Study the drawing (mm; zero at the part's minimum x, y, z) and answer. A direction names the side the tool comes from. Give positions to 0.01 mm unless a question says otherwise; leave off trailing zeros. Write each loop counter-clockwise with the first axis right and the second up, starting at its lowest first coordinate (ties: lowest second). Pieces come first, ordered by that corner, then holes. Notation, with made-up numbers: (66.5, -35) -> (104.5, -35) arc R29 cw to (104.5, -15) -> close; hole circle Ø9 at (-36.5, -9.75). An arc over 180 degrees is marked (long way). One line per question, with ' | ' between items.
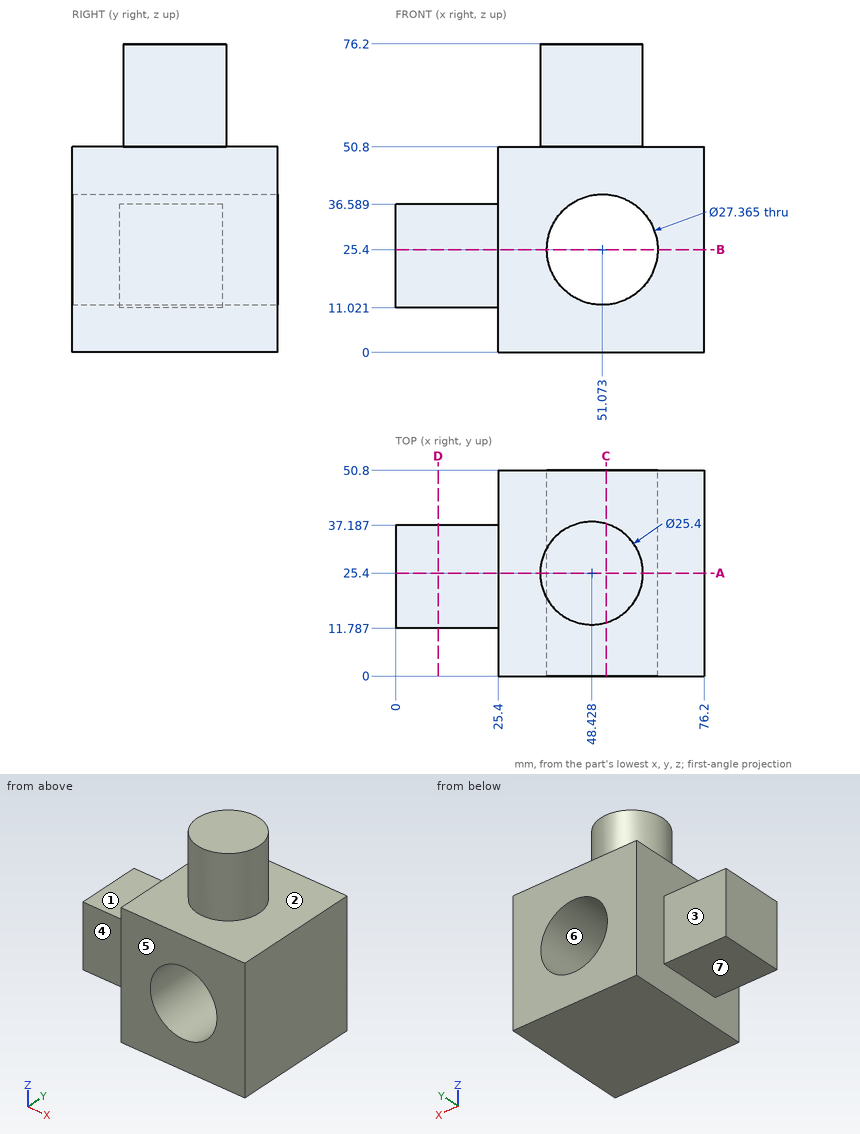
Item 1: Flat-ended cylindrical pins translate along their axes: pin 1 (7.5 mm diameter, centred on x = 7, z = 23, fed in from -Y); pin 2 (2 mm diameter, centred on x = 13.5, y = 10.5, fed in from -Z); pin 3 (12.5 mm diameter, centred on x = 15.5, y = 21, fed in from +Z); pin 4 (1 mm diameter, centred on y = 28, z = 8.5, fed in from -X). Find the tip coordinate at first contact, or state that the pin passes through.
Answers below:
pin 1: y = 11.79 | pin 2: through | pin 3: z = 36.59 | pin 4: x = 25.4
Item 2: Find section A-A (y = 25.4). Write down the section's boundary in (x, z) (1 decimal), then the cut area to 3 significant figures.
Answers below:
outline: (0, 11) -> (25.4, 11) -> (25.4, 0) -> (76.2, 0) -> (76.2, 50.8) -> (61.1, 50.8) -> (61.1, 76.2) -> (35.7, 76.2) -> (35.7, 50.8) -> (25.4, 50.8) -> (25.4, 36.6) -> (0, 36.6) -> close; hole circle Ø27.4 at (51.1, 25.4) | area: 3,290 mm²
Item 3: Determine the mould class of the marked faces 5, 6 and 7 for opening direction Z: pulls with the +Z half, pulls with the -Z half, needs draft (parallel to the pull), parting line crosses it, or undercut.
Answers below:
face 5: needs draft | face 6: undercut | face 7: pulls with the -Z half
Item 4: Find section D-D (x = 10.5). Write down the section's boundary in (y, z).
Answers below:
outline: (11.79, 11.02) -> (37.19, 11.02) -> (37.19, 36.59) -> (11.79, 36.59) -> close
Item 5: Consider line 1 (X direction, y = 28, z = 25); line 2 (Z direction, x = 50.5, y = 46); line 3 (Y direction, x = 17, z = 12). Determine where each line is inside the solid, lowest interval first. Write a range as [from, to].
Answers below:
line 1: [0, 37.4], [64.75, 76.2] | line 2: [0, 11.73], [39.07, 50.8] | line 3: [11.79, 37.19]
Item 6: Find section B-B (z = 25.4). Write down the section's boundary in (x, y) (1 decimal), then the cut area to 3 significant figures.
Answers below:
outline: (0, 11.8) -> (25.4, 11.8) -> (25.4, 0) -> (37.4, 0) -> (37.4, 50.8) -> (25.4, 50.8) -> (25.4, 37.2) -> (0, 37.2) -> close; (64.8, 0) -> (76.2, 0) -> (76.2, 50.8) -> (64.8, 50.8) -> close | area: 1,840 mm²
Item 7: A tool of negligible diameter and unlimited length cuts with its end or side. For the marked faces 1, 2, 3 and 4, from which of +Z, -Z, +X, -X, +Y, -Y can it reach the whole face along a straight path? Write none if from no direction.
Answers below:
face 1: +Z, -X, +Y, -Y | face 2: +Z | face 3: +Z, -Z, -X, +Y | face 4: +Z, -Z, -X, -Y
Item 8: Find section C-C (x = 52). Write down the section's boundary in (y, z).
Answers below:
outline: (0, 0) -> (50.8, 0) -> (50.8, 11.75) -> (0, 11.75) -> close; (0, 39.05) -> (50.8, 39.05) -> (50.8, 50.8) -> (37.59, 50.8) -> (37.59, 76.2) -> (13.21, 76.2) -> (13.21, 50.8) -> (0, 50.8) -> close
